Input: part model. Units: mm. Frame: model coordinates. Round coordinates to 2 decimals unless told otherwise and drop trailing zeros. Order: outer loops, then holes, each group sorted by start corner. A loop starts at its lowest first (then second) coordinate and runs counter-clockwise, first axis right, second up. Notation, with made-up numbers: M 22,18.25 L 44,18.25 A29 cw 44,42.25 Z; hole C 80,38.25 d4. An arc over 180 degrees is marked long. One line per question, with ' | ' between items.
```python
from build123d import *

# Parameters (mm, degrees)
SKETCH1_R           = 5
BOSS_EXTRUDE1_DEPTH = 5


with BuildPart() as part:
    # Sketch1 → Boss-Extrude1 (new body)
    with BuildSketch(Plane.XY):
        with BuildLine():
            Line((-54.933450377, 27.554820012), (15.066549623, 27.554820012))
            ThreePointArc((15.066549623, 27.554820012), (25.066549623, 17.554820012), (15.066549623, 7.554820012))
            Line((15.066549623, 7.554820012), (-54.933450377, 7.554820012))
            ThreePointArc((-54.933450377, 7.554820012), (-64.933450377, 17.554820012), (-54.933450377, 27.554820012))
        make_face()
        with Locations((-54.933450377, 17.554820012)):
            Circle(SKETCH1_R, mode=Mode.SUBTRACT)
        with Locations((15.066549623, 17.554820012)):
            Circle(SKETCH1_R, mode=Mode.SUBTRACT)
    extrude(amount=BOSS_EXTRUDE1_DEPTH)


solid = part.part
```
Item 1: Mould query, pull axis Y, two halves, no side actions, for faces 1 (the cylindrical face through (-64.93, 17.33, 2.46)), 2 (the flat face through (-19, 18, 5)), 3 (the cylindrical face through (19.836, 19.057, 2.465)). Classes: +Y half, -Y half, draft (parallel to the pull), parting line (faces both ways), or undercut.
Report:
face 1: parting line | face 2: draft | face 3: undercut
Item 2: First-contact query: pin 1 (2 mm diameter, centred on y = 12.5, z = 4.5, fed in from -X). Flat tip, straight axial feed; report the tip coordinate or a pass-through.
Report:
pin 1: x = -64.07
Item 3: Section query B-B, the plane x = -52. Return loops of the section in (y, z), plus the area to 3 significant figures.
Report:
outline: M 7.55,0 L 13.51,0 L 13.51,5 L 7.55,5 Z; M 21.6,0 L 27.55,0 L 27.55,5 L 21.6,5 Z | area: 59.5 mm²
Item 4: Section query C-C, the plane z = 2.7. Return loops of the section in (x, y).
Report:
outline: M -54.93,7.55 L 15.07,7.55 A10 ccw 15.07,27.55 L -54.93,27.55 A10 ccw Z; hole C -54.93,17.55 d10; hole C 15.07,17.55 d10
Item 5: Line query: line 1 along X through (y, z) = (17.25, 1.95); line 2 along X through (y, z) = (14, 4.75); line 3 along Y through (x, z) = (15.5, 3.85). Output: solid intervals per line, ascending. Write a range as from..to.
Report:
line 1: -64.93..-59.92, -49.94..10.08, 20.06..25.06 | line 2: -64.28..-58.45, -51.42..11.55, 18.58..24.41 | line 3: 7.56..12.57, 22.54..27.55
Item 6: Section query A-A, the plane y = 21.75. Return loops of the section in (x, z), plus the area to 3 significant figures.
Report:
outline: M -64.01,0 L -57.65,0 L -57.65,5 L -64.01,5 Z; M -52.21,0 L 12.35,0 L 12.35,5 L -52.21,5 Z; M 17.79,0 L 24.14,0 L 24.14,5 L 17.79,5 Z | area: 386 mm²
Item 7: Section query D-D, the plane y = 15.5. Return loops of the section in (x, z).
Report:
outline: M -64.72,0 L -59.49,0 L -59.49,5 L -64.72,5 Z; M -50.38,0 L 10.51,0 L 10.51,5 L -50.38,5 Z; M 19.62,0 L 24.85,0 L 24.85,5 L 19.62,5 Z
